Could you check a few things on this drawing? It's one solid part, dimensions in mm from its lowest x, y, z. Round coordinates to 2 decimals unless told otherwise and drop trailing zeros. Order: outer loops, then holes, each group sorted by start corner. A loop starts at its lowest first (then second) coordinate and runs counter-clockwise, first axis right, second up. Notation, with made-up numbers: M 86.5,-13 L 122.5,-13 A8 cw 122.5,-8 Z; hole C 40,60 d9. An arc over 180 degrees is marked long. Answer as a JSON object with one key per item and string values. Group by question number.
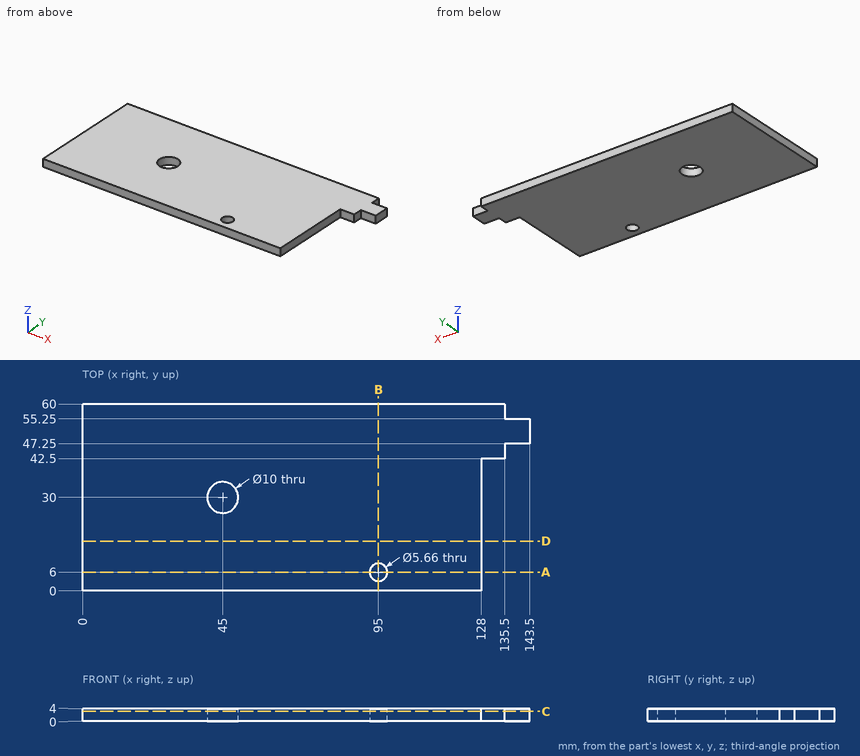
1) If we section it at B-B on x = 95: Write out the boundary of the cut face in (y, z), plus the area to 3 significant figures.
2) If we section it at D-D on y = 16: Write out the boundary of the cut face in (x, z).
3) If we section it at C-C on z = 3.25: Write out the boundary of the cut face in (x, y), plus the area to 3 significant figures.
4) I need wall thicknesses on line 1 along Y through (x, z) = (95, 2.25); line 2 along Y through (x, z) = (45, 2.95); line 3 along X through (y, z) = (39, 2.15). Which ranges of each line are inside material? Lowest first, please.
5) If we section it at A-A on y = 6: Write out the boundary of the cut face in (x, z), plus the area to 3 significant figures.
6) For pin 1 (2 mm diameter, centred on y = 27, z = 2.5, fed in from +X); pin 2 (2 mm diameter, centred on y = 44, z = 1.5, fed in from +X), each with a flat end and sliding along its axis, tell me the tip position at first contact or that it passes through.
Findings:
{
 "1": {"outline": "M 0,0 L 3.17,0 L 3.17,4 L 0,4 Z; M 8.83,0 L 60,0 L 60,4 L 8.83,4 Z", "area": "217 mm^2"},
 "2": {"outline": "M 0,0 L 128,0 L 128,4 L 0,4 Z"},
 "3": {"outline": "M 0,0 L 128,0 L 128,42.5 L 135.5,42.5 L 135.5,47.25 L 143.5,47.25 L 143.5,55.25 L 135.5,55.25 L 135.5,60 L 0,60 Z; hole C 45,30 d10; hole C 95,6 d5.66", "area": "7,770 mm^2"},
 "4": {"line 1": "y = 0 to 3.17, 8.83 to 60", "line 2": "y = 0 to 25, 35 to 60", "line 3": "x = 0 to 128"},
 "5": {"outline": "M 0,0 L 92.17,0 L 92.17,4 L 0,4 Z; M 97.83,0 L 128,0 L 128,4 L 97.83,4 Z", "area": "489 mm^2"},
 "6": {"pin 1": "stops at x = 128", "pin 2": "stops at x = 135.5"}
}
